Could you check a few things on this model? Use its own coordinates, in mm. A direction names the side the tool comes from. Give positions to 0.01 mm unless a question says otherwise; leave off trailing zeros. Order: outer loops, then holes, each group sorted by start corner. A loop starts at its lowest first (then second) coordinate and runs counter-clockwise, first axis right, second up. Notation, with made-up numbers: (53.25, 5.25) - (96.25, 5.25) arc R30 cw to (96.25, 43.25) - close; hole circle Ø1 at (-3, 40.25). An arc over 180 degrees is marked (long way). Put each result on its own line as item: value.
from build123d import *

# Parameters (mm, degrees)
BOSS_EXTRUDE1_DEPTH     = 12.7
SKETCH3_R               = 4.039553008
CUT_EXTRUDE1_DEPTH      = 80.451479119
SKETCH4_R               = 6.227777938
BOSS_EXTRUDE3_DEPTH     = 12.7
SKETCH5_W               = 55.88
SKETCH5_H               = 98.530771833
CUT_EXTRUDE2_DEPTH      = 13.7
CUT_EXTRUDE2_DEPTH_BACK = 13.7
SKETCH6_W               = 55.88
SKETCH6_H               = 15.424799931
CUT_EXTRUDE3_DEPTH      = 10.16
SKETCH7_W               = 60.96
SKETCH7_H               = 103.610771833
BOSS_EXTRUDE4_DEPTH     = 7.62
SKETCH8_W               = 55.88
SKETCH8_H               = 98.530771833
CUT_EXTRUDE4_DEPTH      = 6.35


with BuildPart() as part:
    # Sketch1 → Boss-Extrude1 (new body)
    with BuildSketch(Plane(origin=(0, 0, 0), x_dir=(1, 0, 0), z_dir=(0, 1, 0))):
        with BuildLine():
            Line((-24.894407518, 17.78), (41.145592482, 17.78))
            ThreePointArc((41.145592482, 17.78), (53.717951052, 12.572358569), (58.925592482, 0))
            Line((58.925592482, 0), (41.145592482, 0))
            Line((41.145592482, 0), (41.145592482, -167.64))
            Line((41.145592482, -167.64), (58.925592482, -167.64))
            ThreePointArc((58.925592482, -167.64), (53.717951052, -180.212358569), (41.145592482, -185.42))
            Line((41.145592482, -185.42), (-24.894407518, -185.42))
            ThreePointArc((-24.894407518, -185.42), (-34.577054874, -178.775485757), (-38.305886636, -167.64))
            Line((-38.305886636, -167.64), (-19.814407518, -167.64))
            Line((-19.814407518, -167.64), (-19.814407518, 0))
            Line((-19.814407518, 0), (-38.305886636, 0))
            ThreePointArc((-38.305886636, 0), (-34.577054874, 11.135485757), (-24.894407518, 17.78))
        make_face()
    extrude(amount=BOSS_EXTRUDE1_DEPTH)

    # Sketch3 → Cut-Extrude1 (cut, through all)
    with BuildSketch(Plane(origin=(41.145592482, 0, 0), x_dir=(0, 0, -1), z_dir=(1, 0, 0))):
        with Locations((-139.663754312, 12.7)):
            Circle(SKETCH3_R)
        with Locations((-27.973876463, 12.7)):
            Circle(SKETCH3_R)
    extrude(amount=-CUT_EXTRUDE1_DEPTH, mode=Mode.SUBTRACT)

    # Sketch4 → Boss-Extrude3 (add)
    with BuildSketch(Plane(origin=(0, 12.7, 0), x_dir=(1, 0, 0), z_dir=(0, 1, 0))):
        with Locations((30.41662766, -8.42802752)):
            Circle(SKETCH4_R)
        with Locations((30.41662766, -159.21197248)):
            Circle(SKETCH4_R)
        with Locations((-9.085442695, -159.21197248)):
            Circle(SKETCH4_R)
        with Locations((-9.085442695, -8.42802752)):
            Circle(SKETCH4_R)
    extrude(amount=BOSS_EXTRUDE3_DEPTH)

    # Sketch5 → Cut-Extrude2 (cut, two sides)
    with BuildSketch(Plane(origin=(0, 12.7, 0), x_dir=(1, 0, 0), z_dir=(0, 1, 0))) as cut_extrude2_sk:
        with Locations((10.665592482, -83.818815387)):
            Rectangle(SKETCH5_W, SKETCH5_H)
    extrude(amount=CUT_EXTRUDE2_DEPTH, mode=Mode.SUBTRACT)
    extrude(cut_extrude2_sk.sketch, amount=-CUT_EXTRUDE2_DEPTH_BACK, mode=Mode.SUBTRACT)

    # Sketch6 → Cut-Extrude3 (cut)
    with BuildSketch(Plane(origin=(0, 12.7, 0), x_dir=(1, 0, 0), z_dir=(0, 1, 0))):
        with Locations((10.665592482, -175.814372445)):
            Rectangle(SKETCH6_W, SKETCH6_H)
        with Locations((10.665592482, 8.174372446)):
            Rectangle(SKETCH6_W, SKETCH6_H)
    extrude(amount=-CUT_EXTRUDE3_DEPTH, mode=Mode.SUBTRACT)

    # Sketch7 → Boss-Extrude4 (add)
    with BuildSketch(Plane.XZ):
        with Locations((10.665592482, 83.818815387)):
            Rectangle(SKETCH7_W, SKETCH7_H)
    extrude(amount=BOSS_EXTRUDE4_DEPTH)

    # Sketch8 → Cut-Extrude4 (cut, symmetric)
    with BuildSketch(Plane(origin=(0, 0, 0), x_dir=(1, 0, 0), z_dir=(0, 1, 0))):
        with Locations((10.665592482, -83.818815387)):
            Rectangle(SKETCH8_W, SKETCH8_H)
    extrude(amount=CUT_EXTRUDE4_DEPTH, both=True, mode=Mode.SUBTRACT)


solid = part.part
1) Suppose I cut it at A-A, the plane z = 43. List the corners of the cut face in (x, y) for me.
Filled in:
outline: (-19.81, -7.62) - (41.15, -7.62) - (41.15, 12.7) - (38.61, 12.7) - (38.61, -6.35) - (-17.27, -6.35) - (-17.27, 12.7) - (-19.81, 12.7) - close
2) If I drill on line 1 (Z direction, x = 5.5, y = 5); line 2 (X direction, y = 4, z = 64.5); line 3 (Z direction, x = -9, y = 10.5), over which ranges is the centre line in solid material (lowest first)? Write a range as [from, to].
Filled in:
line 1: z = [-17.78, -15.89], [-0.46, 34.55], [133.08, 168.1], [183.53, 185.42]
line 2: x = [-19.81, -17.27], [38.61, 41.15]
line 3: z = [-17.78, -15.89], [-0.46, 24.59], [31.36, 34.55], [133.08, 136.28], [143.05, 168.1], [183.53, 185.42]
3) Suppose I cut it at D-D, the plane z = 6. List the corners of the cut face in (x, y) for me, and give its area (3 significant figures).
Filled in:
outline: (-19.81, 0) - (41.15, 0) - (41.15, 12.7) - (36.15, 12.7) - (36.15, 25.4) - (24.68, 25.4) - (24.68, 12.7) - (-3.35, 12.7) - (-3.35, 25.4) - (-14.82, 25.4) - (-14.82, 12.7) - (-19.81, 12.7) - close
area: 1,070 mm^2
4) Suppose I cut it at C-C, the plane y = 16. List the corners of the cut face in (x, z) for me.
Filled in:
outline: circle Ø12.46 at (-9.09, 8.43); circle Ø12.46 at (-9.09, 159.21); circle Ø12.46 at (30.42, 8.43); circle Ø12.46 at (30.42, 159.21)
5) Suppose I cut it at B-B, the plane x = 50. List the corners of the cut face in (y, z) for me.
Filled in:
outline: (0, -15.42) - (12.7, -15.42) - (12.7, 0) - (0, 0) - close; (0, 167.64) - (12.7, 167.64) - (12.7, 183.06) - (0, 183.06) - close
6) I'm going to push flat-ended pins straight in: pin 1 (2 mm diameter, centred on x = 3, z = 134.5, fed in from +Y); pin 2 (3 mm diameter, centred on x = 43, y = 3, fed in from -Z); pin 3 (4 mm diameter, centred on x = 6.5, z = 65, fed in from +Y). Where does each tip first touch, or does it pass through?
Filled in:
pin 1: stops at y = 12.7
pin 2: stops at z = -17.78
pin 3: stops at y = -6.35
7) Which directions (+Z, -Z, +X, -X, +Y, -Y) give clear straight access to the entire face, cutting with the end or side of a thin tool? Please do faces 1 (the cylindrical face through (11.09, 8.66, 28.06)), 2 (the flat face through (10, -4, 135.624)), 3 (the flat face through (10, 2.54, -8)).
Filled in:
face 1: +X, -X, +Y
face 2: +Z, +X, -X, -Y
face 3: +Y
8) We'd pull the mould along Z, two halves only. Please class faces 4 (the flat face through (-9, 25.4, 159)), 5 (the flat face through (9, 6, 185.42)), 6 (the flat face through (50, 6, 0)): pulls with the +Z half, pulls with the -Z half, needs draft (parallel to the pull), parting line crosses it, or undercut.
Filled in:
face 4: needs draft
face 5: pulls with the +Z half
face 6: undercut
